For this review, use the dimensioned drawing (mm, ordinates from the lowest corner) and the shaded views. Round coordinates to 2 decimals unless told otherwise and drop trailing zeros. Write each loop counter-clockwise with the first axis right and the second up, starting at its lowest first coordinate (ties: lowest second). Pieces come first, ordered by that corner, then holes. Notation, with made-up numbers: (80, -14.5) -> (104, -14.5) arc R36 cw to (104, 24.5) -> close; hole circle Ø6 at (-23, -12). An arc over 180 degrees is marked (long way). Write each question's results on one line, items separated by ' | '. Start each with the question number.
Item 1: Add section C-C (x = 1513). State the section outline as (y, z) points, plus the area to 3 significant figures.
Item 2: Clearance check with flat-ended pins moving along their axes: pin 1 (6 mm diameter, centred on x = 186, z = 9.5, fed in from +Y); pin 2 (8 mm diameter, centred on y = 130.5, z = 43, fed in from +X); pin 3 (22 mm diameter, centred on x = 972, z = 11, fed in from +Y); pin 4 (15 mm diameter, centred on y = 352, z = 35, fed in from -X). State where each tip first meets the part, or that it passes through.
Item 3: Add section A-A (y = 143). State the section outline as (x, z) points.
Item 4: To check wall thickness, follow line 1 along X through (y, z) = (67.5, 16.5); line 2 along X through (y, z) = (49, 110); line 3 along Y through (x, z) = (1525, 7.5). State the ranges of each line that lie inside material, in increasing order.
Item 5: Add section B-B (x = 194). State the section outline as (y, z) points.
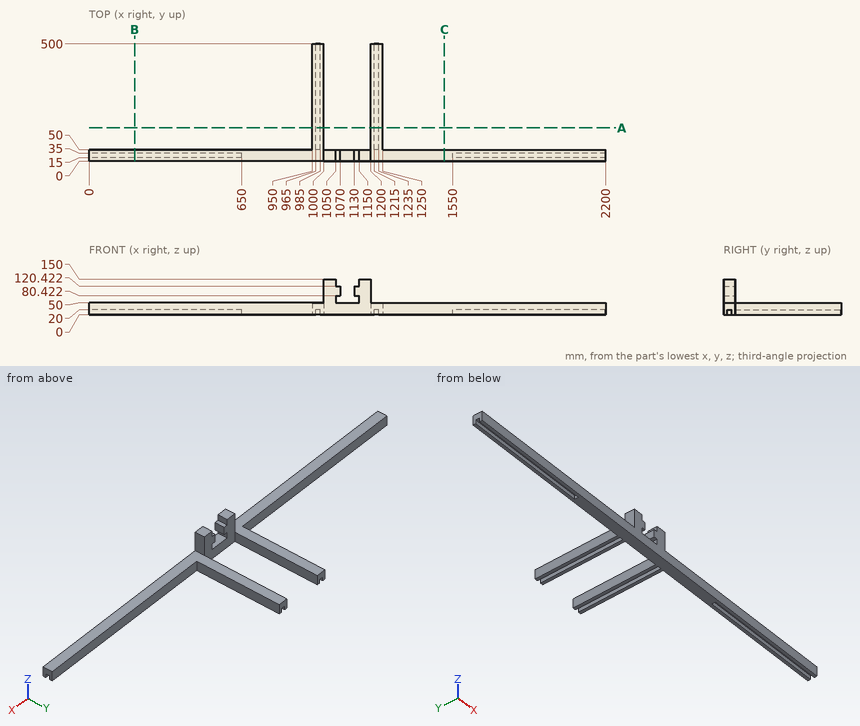
Responses:
1) outline: (0, 0) -> (50, 0) -> (50, 50) -> (0, 50) -> close | area: 2,500 mm^2
2) pin 1: stops at y = 50 | pin 2: stops at x = 1250 | pin 3: stops at y = 500 | pin 4: stops at x = 950
3) outline: (950, 0) -> (965, 0) -> (965, 20) -> (985, 20) -> (985, 0) -> (1000, 0) -> (1000, 50) -> (950, 50) -> close; (1200, 0) -> (1215, 0) -> (1215, 20) -> (1235, 20) -> (1235, 0) -> (1250, 0) -> (1250, 50) -> (1200, 50) -> close
4) line 1: x = 950 to 965, 985 to 1000, 1200 to 1215, 1235 to 1250 | line 2: x = 1000 to 1070, 1130 to 1200 | line 3: y = 0 to 50
5) outline: (0, 0) -> (15, 0) -> (15, 20) -> (35, 20) -> (35, 0) -> (50, 0) -> (50, 50) -> (0, 50) -> close
